Model file for the job. Use its own axes, mm. A direction names the side the tool comes from. Round coordinates to 2 decimals unless told otherwise and drop trailing zeros. Loops run counter-clockwise (first coordinate to the right, second up) from the corner with the lowest first, then second, coordinate; pieces in that order, holes last. Notation, with made-up numbers: M 41.5,26 L 86.5,26 A19 cw 86.5,31 Z; hole C 16,-4 d11. An arc over 180 degrees is marked long. Answer in a Markdown table with one row per item.
Autodesk Inventor part; units mm, degrees
ref_plane "YZ Plane" through (0, 0, 0) normal (1, 0, 0) x (0, 1, 0)
ref_plane "XZ Plane" through (0, 0, 0) normal (0, 1, 0) x (-1, 0, 0)
ref_plane "XY Plane" through (0, 0, 0) normal (0, 0, 1) x (1, 0, 0)
sketch "Sketch1" plane through (0, 0, 0) normal (0, 0, 1) x (1, 0, 0)
  line L0 (-1.6732, 2.8981) -> (1.6732, 2.8981)
  line L1 (-3.3464, 0) -> (-1.6732, 2.8981)
  line L2 (-1.6732, -2.8981) -> (-3.3464, 0)
  line L3 (1.6732, -2.8981) -> (-1.6732, -2.8981)
  line L4 (3.3464, 0) -> (1.6732, -2.8981)
  line L5 (1.6732, 2.8981) -> (3.3464, 0)
  line L6 (3.0288, 4.8981) -> (5.8567, 0)
  line L7 (-2.627, 4.8981) -> (3.0288, 4.8981)
  line L8 (-5.4549, 0) -> (-2.627, 4.8981)
  line L9 (-2.627, -4.8981) -> (-5.4549, 0)
  line L10 (3.0288, -4.8981) -> (-2.627, -4.8981)
  line L11 (5.8567, 0) -> (3.0288, -4.8981)
  point P0 (0, 0)
extrude "Extrusion1" add sketch "Sketch1" against normal blind 10
sketch "Sketch2" plane through (0, 0, 0) normal (0, 0, 1) x (1, 0, 0)
  line L0 (3.0288, 4.8981) -> (-2.627, 4.8981)
  line L1 (-2.627, 4.8981) -> (-5.4549, 0)
  line L2 (-5.4549, 0) -> (-2.627, -4.8981)
  line L3 (-2.627, -4.8981) -> (3.0288, -4.8981)
  line L4 (3.0288, -4.8981) -> (5.8567, 0)
  line L5 (5.8567, 0) -> (3.0288, 4.8981)
  point P0 (0, 0)
extrude "Extrusion2" add sketch "Sketch2" along normal blind 3
sketch "Sketch3" plane through (0, 0, 3) normal (0, 0, 1) x (1, 0, 0)
  circle A0 centre (0, 0) radius 4
  circle A1 centre (0, 0) radius 2.275
  dimension "d4" = 8
  dimension "d5" = 4.55
extrude "Extrusion3" add sketch "Sketch3" along normal blind 10
fillet "Fillet1" radius 1 1 edges at (-4, 0, 3)
sketch "Sketch4" plane through (-2.627, 4.8981, -10) normal (0, 1, 0) x (1, 0, 0)
  line L0 (5.6558, 0) -> (5.6558, -13)
  line L1 (0, 0) -> (5.6558, 0)
  line L2 (0, -13) -> (0, 0)
  line L3 (5.6558, -13) -> (3.6314, -13)
  line L4 (0.9538, -10) -> (4.3002, -10)
  line L5 (5.6558, 0) -> (0, 0)
  line L6 (2.8279, 0) -> (2.8279, -10) construction
  circle A0 centre (2.8279, -5.002) radius 0.625
  line L7 (1.6226, -13) -> (0, -13)
  point P0 (2.627, -10)
  point P1 (2.8279, 0)
  dimension "d9" = 1.25
extrude "Extrusion4" cut sketch "Sketch4" against normal blind 10
properties part number "Acople_Motor"
1. Mould opens along X. For faces 6 (the flat face through (-1, -2.898, -5)), 7 (the flat face through (0, -4.898, -3)), 8 (the flat face through (-4.021, -2.483, -3.389)) say: +X half, -X half, draft (parallel to the pull), parting line (faces both ways), or undercut.
Verdict:
| item | result |
|---|---|
| face 6 | undercut |
| face 7 | draft |
| face 8 | -X half |
2. Saw through at B-B (x = 0). Write the cut outline in (y, z) (3 decimals).
Verdict:
| item | result |
|---|---|
| outline | M -4.898,-10 L -2.898,-10 L -2.898,-5.59 L -4.898,-5.59 Z; M -4.898,-4.406 L -2.898,-4.406 L -2.898,0 L 2.898,0 L 2.898,-4.406 L 4.898,-4.406 L 4.898,3.005 A1 cw 4,4 L 4,13 L 2.275,13 L 2.275,3 L -2.275,3 L -2.275,13 L -4,13 L -4,4 A1 cw -4.898,3.005 Z; M 2.898,-10 L 4.898,-10 L 4.898,-5.59 L 2.898,-5.59 Z |
3. Tool access for faces 1 (the cylindrical face through (-0.867, 3.905, 8.437)), 2 (the flat face through (-2.4, -4.6, 3)), 3 (the flat face through (5.2, 0, 3)), 4 (the flat face through (2.52, -1.43, -4.93)), 5 (the flat face through (-2.4, 4.6, 3)): list every direction of +Z, -Z, +X, -X, +Y, -Y with a clear straight run to the whole face (end or side of a thin tool).
Verdict:
| item | result |
|---|---|
| face 1 | +Z |
| face 2 | +Z, -X, -Y |
| face 3 | +Z, +X |
| face 4 | -Z |
| face 5 | +Z, -X, +Y |
4. Saw through at C-C (z = 4.5). Write the cut outline in (x, y) (3 decimals).
Verdict:
| item | result |
|---|---|
| outline | C 0,0 d8; hole C 0,0 d4.55 |
5. Pin check, flat tips, straight feed: pin 1 (0.6 mm diameter, centred on x = -2.5, y = -4.5, fed in from +Z); pin 2 (3 mm diameter, centred on x = 1, z = 8.5, fed in from -Y); pin 3 (0.9 mm diameter, centred on x = -2, y = 4.5, fed in from +Z). Stop position of each tip, or through.
Verdict:
| item | result |
|---|---|
| pin 1 | stops at z = 3.01 |
| pin 2 | stops at y = -4 |
| pin 3 | stops at z = 3.15 |
6. Saw through at A-A (z = -0.75). Write the cut outline in (x, y).
Verdict:
| item | result |
|---|---|
| outline | M -5.45,0 L -2.63,-4.9 L 3.03,-4.9 L 5.86,0 L 3.03,4.9 L -2.63,4.9 Z; hole M -3.35,0 L -1.67,-2.9 L 1.67,-2.9 L 3.35,0 L 1.67,2.9 L -1.67,2.9 Z |
7. Wall check: probe 1 along Y at (x, z) = (0, 9.75) (3 decimals); probe 2 along Y at (x, z) = (-0.5, -3.5); probe 3 along Z at (x, y) = (1, 1). Give the ranges that are in metal, low to high.
Verdict:
| item | result |
|---|---|
| probe 1 | y = -4 to -2.275, 2.275 to 4 |
| probe 2 | y = -4.9 to -2.9, 2.9 to 4.9 |
| probe 3 | z = 0 to 3 |
8. Saw through at D-D (x = 5.25). Write the cut outline in (y, z).
Verdict:
| item | result |
|---|---|
| outline | M -1.05,-10 L 1.05,-10 L 1.05,3 L -1.05,3 Z |
